Design review of the part built by this model. Coordinates are the model's own, in mm. A direction names the side the tool comes from. Coordinates: 2 decimals unless noted, no trailing zeros. Loops run counter-clockwise (first coordinate to the right, second up) from the corner with the lowest first, then second, coordinate; pieces in that order, holes last. Notation, with made-up numbers: (-32.5, -7.75) -> (14.5, -7.75) arc R19 cw to (14.5, 23.25) -> close; hole circle Ø1 at (25.5, 6). An arc over 180 degrees is marked (long way). Use a Markdown table: item, result. Add a question column.
Q1. Take a section at B-B on z = 0.4. Write out the cut boundary in (x, y).
Q2. Draft analysis for pull direction X (two halves, no side actions). For faces 1 (the face through (-6, 25, 0)), 2 (the face through (2, -2, 4.5)), 3 (the face through (-0.46, 47.95, 0.02)), state which applies: pulls with the +X half, pulls with the -X half, needs draft (parallel to the pull), parting line crosses it, or undercut.
Q3. Take a section at D-D on z = 2.7. Write out the cut boundary in (x, y), plus the area to 3 significant figures.
Q4. Take a section at A-A on x = 0. Write out the cut boundary in (y, z), plus the area to 3 significant figures.
Q5. For faces 4 (the face through (-1.08, -4.88, 2.98)), 5 (the face through (0, -6, 0)), list the 3-axis set-ups (+Z, -Z, +X, -X, +Y, -Y) from which the entire face can be reached by the end or side of a thin tool; tool diameter is ignored.
Q6. Clearance check with flat-ended pins moving along their axes: pin 1 Ø5 at (x, y) = (0, 50) entering from +Z; pin 2 Ø6 at (x, y) = (0, 0) entering from +Z. State where each tip first meets the part, or that it passes through.
Q7. For probe 1 along Y at (x, z) = (0, 0.9); probe 2 along Y at (x, z) = (-1.25, 1.4); probe 3 along Z at (x, y) = (3.5, 6), list the stretches that pass through material, from the lowest coordinate up.
Q8. Take a section at C-C on y = 51.5. Write out the cut boundary in (x, z), plus the area to 3 significant figures.
from build123d import *

# Parameters (mm, degrees)
BOSS_EXTRUDE1_DEPTH = 1.5
SKETCH2_R           = 5
SKETCH2_R_2         = 2.5
BOSS_EXTRUDE2_DEPTH = 3
CUT_EXTRUDE1_REACH  = 58.4
SKETCH2_2_R         = 2.5
CUT_EXTRUDE2_REACH  = 58.4
SKETCH5_R           = 2.1


with BuildPart() as part:
    # Sketch1 → Boss-Extrude1 (new, symmetric)
    with BuildSketch(Plane.XY):
        with BuildLine():
            Line((-6, 50), (-6, 0))
            ThreePointArc((-6, 0), (0, -6), (6, 0))
            Line((6, 0), (6, 50))
            ThreePointArc((6, 50), (0, 56), (-6, 50))
        make_face()
    extrude(amount=BOSS_EXTRUDE1_DEPTH, both=True)

    # Sketch2 → Boss-Extrude2 (add)
    with BuildSketch(Plane.XY.offset(1.5)):
        Circle(SKETCH2_R)
        Circle(SKETCH2_R_2, mode=Mode.SUBTRACT)
    extrude(amount=BOSS_EXTRUDE2_DEPTH)

    # Sketch2<2> → Cut-Extrude1 (cut, up to next)
    with BuildSketch(Plane.XY.offset(1.5), mode=Mode.PRIVATE) as cut_extrude1_sk1:
        Circle(SKETCH2_2_R)
    cut_extrude1_tool1 = extrude(cut_extrude1_sk1.sketch, amount=-CUT_EXTRUDE1_REACH, mode=Mode.PRIVATE) & part.part
    add(cut_extrude1_tool1.solids().sort_by_distance((0, 0, 1.5))[0], mode=Mode.SUBTRACT)

    # Sketch5 → Cut-Extrude2 (cut, up to next)
    with BuildSketch(Plane.XY.offset(1.5), mode=Mode.PRIVATE) as cut_extrude2_sk1:
        with Locations((0, 50)):
            Circle(SKETCH5_R)
    cut_extrude2_tool1 = extrude(cut_extrude2_sk1.sketch, amount=-CUT_EXTRUDE2_REACH, mode=Mode.PRIVATE) & part.part
    add(cut_extrude2_tool1.solids().sort_by_distance((0, 50, 1.5))[0], mode=Mode.SUBTRACT)


solid = part.part
Answer list:
| question | item | result |
|---|---|---|
| 1 | outline | (-6, 0) arc R6 ccw to (6, 0) -> (6, 50) arc R6 ccw to (-6, 50) -> close; hole circle Ø5 at (0, 0); hole circle Ø4.2 at (0, 50) |
| 2 | face 1 | pulls with the -X half |
| 2 | face 2 | needs draft |
| 2 | face 3 | undercut |
| 3 | outline | circle Ø10 at (0, 0); hole circle Ø5 at (0, 0) |
| 3 | area | 58.9 mm² |
| 4 | outline | (-6, -1.5) -> (-2.5, -1.5) -> (-2.5, 4.5) -> (-5, 4.5) -> (-5, 1.5) -> (-6, 1.5) -> close; (2.5, -1.5) -> (47.9, -1.5) -> (47.9, 1.5) -> (5, 1.5) -> (5, 4.5) -> (2.5, 4.5) -> close; (52.1, -1.5) -> (56, -1.5) -> (56, 1.5) -> (52.1, 1.5) -> close |
| 4 | area | 173 mm² |
| 5 | face 4 | +Z |
| 5 | face 5 | +Z, -Z, -Y |
| 6 | pin 1 | z = 1.5 |
| 6 | pin 2 | z = 4.5 |
| 7 | probe 1 | -6 to -2.5, 2.5 to 47.9, 52.1 to 56 |
| 7 | probe 2 | -5.87 to -2.17, 2.17 to 48.31, 51.69 to 55.87 |
| 7 | probe 3 | -1.5 to 1.5 |
| 8 | outline | (-5.81, -1.5) -> (-1.47, -1.5) -> (-1.47, 1.5) -> (-5.81, 1.5) -> close; (1.47, -1.5) -> (5.81, -1.5) -> (5.81, 1.5) -> (1.47, 1.5) -> close |
| 8 | area | 26.0 mm² |
